```python
from build123d import *

# Parameters (mm, degrees)
F1_ANGLE = 10


with BuildPart() as f1:
    # F0 (on Front) → F1 (revolve, symmetric)
    with BuildSketch(Plane.XZ) as f1_sk:
        with BuildLine():
            Line((39.630951, -16.612617), (41.630951, -18))
            add(Edge.make_bspline(
                [(41.630951, -18), (48.621444, -11.169093), (49.786527, -3)],
                knots=[5.696209, 5.696209, 5.696209, 6.190746, 6.190746, 6.190746], degree=2, weights=[1, 0.969585, 1]))
            Line((49.786527, -3), (46.786527, -2))
            Line((46.786527, -2), (46.786527, 4))
            Line((46.786527, 4), (44.786527, 4))
            Line((44.786527, 4), (44.786527, -3))
            Line((44.786527, -3), (47.686527, -5))
            Line((47.686527, -5), (43.658739, -10.806308))
            Line((43.658739, -10.806308), (39.630951, -16.612617))
        make_face()
    revolve(axis=Axis((0, 0, 2.169164), (0, 0, -1)), revolution_arc=F1_ANGLE / 2)
    revolve(f1_sk.sketch, axis=Axis((0, 0, 2.169164), (0, 0, 1)), revolution_arc=F1_ANGLE / 2)


solid = f1.part
```
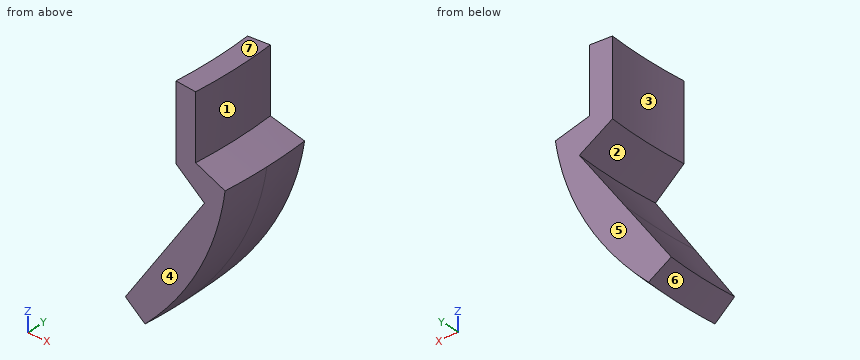
Here's how the part is built. I have some questions about the finished solid (model axes, mm). Face numbers are marked on the shaded views. A direction names the side the tool comes from. Coordinates: 2 decimals unless noted, no trailing zeros. Order: outer loops, then holes, each group sorted by start corner. A loop starts at its lowest first (then second) coordinate and runs counter-clockwise, first axis right, second up. Notation, with made-up numbers: (56, -23.5) - (86, -23.5) arc R23 cw to (86, 3.5) - close; hole circle Ø2 at (32.5, 74.25). An arc over 180 degrees is marked (long way). One line per question, with ' | ' between items. Start each with the question number.
1. If we section it at A-A (z = 2.25): Write out the boundary of the cut face in (x, y), and give its area (3 significant figures).
2. I'm going to push flat-ended pins straight in: pin 1 Ø3 at (x, z) = (44, -3.5) entering from +Y; pin 2 Ø4 at (x, z) = (40.5, -14) entering from +Y; pin 3 Ø1.5 at (x, z) = (45.5, -4) entering from -Y. Where does each tip first touch, or does it pass through?
3. If we mould it in two halves opening along Y, with no side actions, what happens to the marked faces 4, 5, 6 and 7? For each: released by +Y, released by -Y, zero draft, split by the parting line, or undercut.
4. Please list where these lines run through material, in increasing order: line 1 along Z through (x, y) = (47, 0.25); line 2 along Z through (x, y) = (46.5, -3.25); line 3 along Z through (x, y) = (43.75, -1.5). Write a range as [from, to].
5. Which directions (+Z, -Z, +X, -X, +Y, -Y) give clear straight access to the entire face, cutting with the end or side of a thin tool? Please do the marked faces 1, 2 and 3.
Model answer:
1) outline: (44.62, -3.9) - (46.61, -4.08) arc R46.79 ccw to (46.61, 4.08) - (44.62, 3.9) arc R44.79 cw to start | area: 16.0 mm²
2) pin 1: stops at y = 3.98 | pin 2: stops at y = 3.72 | pin 3: stops at y = -4.05
3) face 4: released by -Y | face 5: released by +Y | face 6: undercut | face 7: zero draft
4) line 1: z = [-11.09, -5.99], [-4.53, -2.07] | line 2: z = [-11.76, -6.55], [-4.26, 4] | line 3: z = [-15.7, -10.64]
5) face 1: +Z, +X | face 2: -X | face 3: +Z, -X
